Check sheet for the modelled part. Datum: model origin and axes. Units: mm. A direction names the side the tool comes from. Round coordinates to 2 decimals unless told otherwise and drop trailing zeros. Loops run counter-clockwise (first coordinate to the right, second up) from the corner with the lowest first, then second, coordinate; pieces in that order, holes last. Notation, with made-up numbers: (63, 44) - (117, 44) arc R36 ccw to (117, 81) - close; hole circle Ø10 at (-12.5, 89). An arc over 180 degrees is marked (long way). Answer in a Markdown table with one row per item. Add a question column.
(1) Access from +Z, -Z, +X, -X, +Y, -Y to the whole of each face (thin tool, end or side, straight path). Record for faces 5 (the flat face through (12, -5, 32.5)), 6 (the flat face through (11, -1, 27.5)), 7 (the flat face through (32.5, -5, 0)), 8 (the flat face through (-11, -9, 0)).
(2) Cross-section at C-C on y = -5.5. Enter the section's corners in (x, z).
(3) Cross-section at B-B on z = 0. Enter the section's corners in (x, y).
(4) Cross-section at D-D on y = 2.5. Enter the section's corners in (x, z) (3 decimals), then the cut area to 3 significant figures.
(5) Thickness scan on line 1 along Z through (x, y) = (37.5, 2) (3 decimals); line 2 along Z through (x, y) = (5.28, -8.5) (3 decimals); line 3 along Z through (x, y) = (28, -7.25). Record the ranges inside material, lowest first.
(6) Cross-section at A-A on x = 5.28. Enter the section's corners in (y, z) (3 decimals).
(7) Gauge pin test, flat ends, axial feed: pin 1 (2.5 mm diameter, centred on x = 10, y = -8, fed in from +Z); pin 2 (2.5 mm diameter, centred on x = 12.5, y = -9, fed in from -Z); pin 3 (0.9 mm diameter, centred on y = -8, z = 2, fed in from +X). Record the tip position at first contact, or that the pin passes through.
(8) Mould release check, pull along X, two halves, no side actions. Record for faces 1 (the flat face through (-17, -7, 0)), 2 (the cylindrical face through (-33.27, 2.46, 25.29)), 3 (the flat face through (-1, 5, 31)), 4 (the flat face through (-42.5, 2, 0)): +X half, -X half, draft (parallel to the pull), parting line (faces both ways), or undercut.
from build123d import *

# Parameters (mm, degrees)
CROQUIS1_W              = 85
CROQUIS1_H              = 70
SALIENTE_EXTRUIR1_DEPTH = 5
SALIENTE_EXTRUIR2_DEPTH = 10
CORTAR_EXTRUIR1_DEPTH   = 12
CROQUIS6_W              = 40.5
CROQUIS6_H              = 29.4
CORTAR_EXTRUIR2_DEPTH   = 16
CROQUIS7_R              = 1.435
CORTAR_EXTRUIR3_DEPTH   = 16
CROQUIS8_R              = 1.435
CORTAR_EXTRUIR4_DEPTH   = 6


with BuildPart() as part:
    # Croquis1 → Saliente-Extruir1 (new body)
    with BuildSketch(Plane(origin=(0, 0, 0), x_dir=(1, 0, 0), z_dir=(0, 1, 0))):
        Rectangle(CROQUIS1_W, CROQUIS1_H)
    extrude(amount=SALIENTE_EXTRUIR1_DEPTH)

    # Croquis3 → Saliente-Extruir2 (add)
    with BuildSketch(Plane(origin=(0, 0, 0), x_dir=(-1, 0, 0), z_dir=(0, -1, 0))):
        with BuildLine():
            Line((8.5, 32.5), (-32.5, 32.5))
            Line((-32.5, 32.5), (-32.5, -32.5))
            Line((-32.5, -32.5), (8.5, -32.5))
            ThreePointArc((8.5, -32.5), (41, 0), (8.5, 32.5))
        make_face()
    extrude(amount=SALIENTE_EXTRUIR2_DEPTH)

    # Croquis4 → Cortar-Extruir1 (cut)
    with BuildSketch(Plane(origin=(0, 5, 0), x_dir=(1, 0, 0), z_dir=(0, 1, 0))):
        with BuildLine():
            Line((-8.5, 27.5), (29.5, 27.5))
            Line((29.5, 27.5), (29.5, -27.5))
            Line((29.5, -27.5), (-8.5, -27.5))
            ThreePointArc((-8.5, -27.5), (-36, 0), (-8.5, 27.5))
        make_face()
    extrude(amount=-CORTAR_EXTRUIR1_DEPTH, mode=Mode.SUBTRACT)

    # Croquis6 → Cortar-Extruir2 (cut, through all)
    with BuildSketch(Plane.XZ.offset(10)):
        with Locations((9.25, 0)):
            Rectangle(CROQUIS6_W, CROQUIS6_H)
    extrude(amount=-CORTAR_EXTRUIR2_DEPTH, mode=Mode.SUBTRACT)

    # Croquis7 → Cortar-Extruir3 (cut, through all)
    with BuildSketch(Plane(origin=(0, -10, 0), x_dir=(-1, 0, 0), z_dir=(0, -1, 0))):
        with Locations((-5.28, -20)):
            Circle(CROQUIS7_R)
        with Locations((-5.28, 20)):
            Circle(CROQUIS7_R)
    extrude(amount=-CORTAR_EXTRUIR3_DEPTH, mode=Mode.SUBTRACT)

    # Croquis8 → Cortar-Extruir4 (cut, through all)
    with BuildSketch(Plane(origin=(0, 0, 0), x_dir=(-1, 0, 0), z_dir=(0, -1, 0))):
        with Locations((32.5, -26.5)):
            Circle(CROQUIS8_R)
        with Locations((-37.5, -26.5)):
            Circle(CROQUIS8_R)
        with Locations((-37.5, 26.5)):
            Circle(CROQUIS8_R)
        with Locations((32.5, 26.5)):
            Circle(CROQUIS8_R)
    extrude(amount=-CORTAR_EXTRUIR4_DEPTH, mode=Mode.SUBTRACT)


solid = part.part
Answers:
| question | item | result |
|---|---|---|
| 1 | face 5 | +Z, +X, -X, -Y |
| 1 | face 6 | +Y |
| 1 | face 7 | +Z, -Z, +X, -Y |
| 1 | face 8 | +Y, -Y |
| 2 | outline | (-8.5, -32.5) - (32.5, -32.5) - (32.5, 32.5) - (-8.5, 32.5) arc R32.5 ccw to start; hole (-8.5, -27.5) - (29.5, -27.5) - (29.5, 27.5) - (-8.5, 27.5) arc R27.5 ccw to start |
| 3 | outline | (-42.5, 0) - (-41, 0) - (-41, -10) - (-11, -10) - (-11, -7) - (-36, -7) - (-36, 5) - (-42.5, 5) - close; (29.5, -10) - (32.5, -10) - (32.5, 0) - (42.5, 0) - (42.5, 5) - (29.5, 5) - close |
| 4 | outline | (-42.5, -35) - (42.5, -35) - (42.5, 35) - (-42.5, 35) - close; hole circle Ø2.87 at (-32.5, -26.5); hole circle Ø2.87 at (-32.5, 26.5); hole (-8.5, -27.5) - (29.5, -27.5) - (29.5, 27.5) - (-8.5, 27.5) arc R27.5 ccw to start; hole circle Ø2.87 at (37.5, -26.5); hole circle Ø2.87 at (37.5, 26.5) |
| 4 | area | 2,650 mm^2 |
| 5 | line 1 | z = -35 to -27.935, -25.065 to 25.065, 27.935 to 35 |
| 5 | line 2 | z = -32.5 to -21.435, -18.565 to -14.7, 14.7 to 18.565, 21.435 to 32.5 |
| 5 | line 3 | z = -32.5 to -14.7, 14.7 to 32.5 |
| 6 | outline | (-10, -32.5) - (0, -32.5) - (0, -35) - (5, -35) - (5, -27.5) - (-7, -27.5) - (-7, -21.435) - (-10, -21.435) - close; (-10, -18.565) - (-7, -18.565) - (-7, -14.7) - (-10, -14.7) - close; (-10, 14.7) - (-7, 14.7) - (-7, 18.565) - (-10, 18.565) - close; (-10, 21.435) - (-7, 21.435) - (-7, 27.5) - (5, 27.5) - (5, 35) - (0, 35) - (0, 32.5) - (-10, 32.5) - close |
| 7 | pin 1 | stops at z = 32.5 |
| 7 | pin 2 | stops at z = -32.5 |
| 7 | pin 3 | stops at x = 32.5 |
| 8 | face 1 | undercut |
| 8 | face 2 | undercut |
| 8 | face 3 | draft |
| 8 | face 4 | -X half |
